from build123d import *

# Parameters (mm, degrees)
F0_W      = 31.75
F0_H      = 31.75
F1_DEPTH  = 60.33
F2_W      = 22.23
F2_H      = 22.23
F3_DEPTH  = 6.35
F4_W      = 31.75
F4_H      = 31.75
F5_DEPTH  = 112.71
F6_W      = 22.23
F6_H      = 22.23
F7_DEPTH  = 6.35
F8_W      = 31.75
F8_H      = 31.75
F8_W_2    = 22.23
F8_H_2    = 22.23
F9_DEPTH  = 112.71
F10_W     = 22.23
F10_H     = 22.23
F11_DEPTH = 6.35
F12_W     = 31.75
F12_H     = 31.75
F12_W_2   = 22.23
F12_H_2   = 22.23
F13_DEPTH = 112.71
F14_W     = 22.23
F14_H     = 22.23
F15_DEPTH = 6.35
F16_W     = 31.75
F16_H     = 31.75
F17_DEPTH = 112.71
F18_W     = 22.23
F18_H     = 22.23
F19_DEPTH = 6.35
F20_W     = 31.75
F20_H     = 31.75
F20_W_2   = 22.23
F20_H_2   = 22.23
F21_DEPTH = 112.71
F22_W     = 22.23
F22_H     = 22.23
F23_DEPTH = 6.35
F24_W     = 31.75
F24_H     = 31.75
F24_W_2   = 22.23
F24_H_2   = 22.23
F25_DEPTH = 25.4
F26_W     = 22.23
F26_H     = 22.23
F27_DEPTH = 6.35
F28_W     = 31.75
F28_H     = 31.75
F28_W_2   = 22.23
F28_H_2   = 22.23
F29_DEPTH = 31.75
F32_DEPTH = 12.7
F34_DEPTH = 12.7
F36_DEPTH = 12.7
F38_DEPTH = 12.7
F40_DEPTH = 12.7
F41_W     = 12.7
F41_H     = 12.7
F42_DEPTH = 736.6
F43_DEPTH = 6.35


with BuildPart() as f1:
    # F0 (on Top) → F1 (new body)
    with BuildSketch(Plane.XY):
        with Locations((15.875, 15.875)):
            Rectangle(F0_W, F0_H)
    extrude(amount=F1_DEPTH)

    # F2 (on face) → F3 (join)
    with BuildSketch(Plane.XY.offset(60.33)):
        with Locations((15.875, 15.875)):
            Rectangle(F2_W, F2_H)
    extrude(amount=F3_DEPTH)

    # F4 (on face) → F5 (join)
    with BuildSketch(Plane.XY.offset(66.68)):
        with Locations((15.875, 15.875)):
            Rectangle(F4_W, F4_H)
    extrude(amount=F5_DEPTH)

    # F6 (on face) → F7 (join)
    with BuildSketch(Plane.XY.offset(179.39)):
        with Locations((15.875, 15.875)):
            Rectangle(F6_W, F6_H)
    extrude(amount=F7_DEPTH)

    # F8 (on face) → F9 (join)
    with BuildSketch(Plane.XY.offset(185.74)):
        with Locations((15.875, 15.875)):
            Rectangle(F8_W, F8_H)
        with Locations((15.875, 15.875)):
            Rectangle(F8_W_2, F8_H_2, mode=Mode.SUBTRACT)
        with Locations((15.875, 15.875)):
            Rectangle(F8_W_2, F8_H_2)
    extrude(amount=F9_DEPTH)

    # F10 (on face) → F11 (join)
    with BuildSketch(Plane.XY.offset(298.45)):
        with Locations((15.875, 15.875)):
            Rectangle(F10_W, F10_H)
    extrude(amount=F11_DEPTH)

    # F12 (on face) → F13 (join)
    with BuildSketch(Plane.XY.offset(304.8)):
        with Locations((15.875, 15.875)):
            Rectangle(F12_W, F12_H)
        with Locations((15.875, 15.875)):
            Rectangle(F12_W_2, F12_H_2, mode=Mode.SUBTRACT)
        with Locations((15.875, 15.875)):
            Rectangle(F12_W_2, F12_H_2)
    extrude(amount=F13_DEPTH)

    # F14 (on face) → F15 (join)
    with BuildSketch(Plane.XY.offset(417.51)):
        with Locations((15.875, 15.875)):
            Rectangle(F14_W, F14_H)
    extrude(amount=F15_DEPTH)

    # F16 (on face) → F17 (join)
    with BuildSketch(Plane.XY.offset(423.86)):
        with Locations((15.875, 15.875)):
            Rectangle(F16_W, F16_H)
    extrude(amount=F17_DEPTH)

    # F18 (on face) → F19 (join)
    with BuildSketch(Plane.XY.offset(536.57)):
        with Locations((15.875, 15.875)):
            Rectangle(F18_W, F18_H)
    extrude(amount=F19_DEPTH)

    # F20 (on face) → F21 (join)
    with BuildSketch(Plane.XY.offset(542.92)):
        with Locations((15.875, 15.875)):
            Rectangle(F20_W, F20_H)
        with Locations((15.875, 15.875)):
            Rectangle(F20_W_2, F20_H_2, mode=Mode.SUBTRACT)
        with Locations((15.875, 15.875)):
            Rectangle(F20_W_2, F20_H_2)
    extrude(amount=F21_DEPTH)

    # F22 (on face) → F23 (join)
    with BuildSketch(Plane.XY.offset(655.63)):
        with Locations((15.875, 15.875)):
            Rectangle(F22_W, F22_H)
    extrude(amount=F23_DEPTH)

    # F24 (on face) → F25 (join)
    with BuildSketch(Plane.XY.offset(661.98)):
        with Locations((15.875, 15.875)):
            Rectangle(F24_W, F24_H)
        with Locations((15.875, 15.875)):
            Rectangle(F24_W_2, F24_H_2, mode=Mode.SUBTRACT)
        with Locations((15.875, 15.875)):
            Rectangle(F24_W_2, F24_H_2)
    extrude(amount=F25_DEPTH)

    # F26 (on face) → F27 (join)
    with BuildSketch(Plane.XY.offset(687.38)):
        with Locations((15.875, 15.875)):
            Rectangle(F26_W, F26_H)
    extrude(amount=F27_DEPTH)

    # F28 (on face) → F29 (join)
    with BuildSketch(Plane.XY.offset(693.73)):
        with Locations((15.875, 15.875)):
            Rectangle(F28_W, F28_H)
        with Locations((15.875, 15.875)):
            Rectangle(F28_W_2, F28_H_2, mode=Mode.SUBTRACT)
        with Locations((15.875, 15.875)):
            Rectangle(F28_W_2, F28_H_2)
    extrude(amount=F29_DEPTH)

    # F31 (on face) → F32 (cut)
    with BuildSketch(Plane.XZ):
        with BuildLine():
            Line((15.875, 123.035), (20.64, 123.035))
            ThreePointArc((20.64, 123.035), (12.5056361876, 126.4043638124), (15.875, 118.27))
            Line((15.875, 118.27), (15.875, 123.035))
        make_face()
        with BuildLine():
            ThreePointArc((15.875, 118.27), (19.2443638124, 119.6656361876), (20.64, 123.035))
            Line((20.64, 123.035), (15.875, 123.035))
            Line((15.875, 123.035), (15.875, 118.27))
        make_face()
    extrude(amount=-F32_DEPTH, mode=Mode.SUBTRACT)

    # F33 (on face) → F34 (cut)
    with BuildSketch(Plane.YZ.offset(31.75)):
        with BuildLine():
            Line((15.875, 242.095), (20.64, 242.095))
            ThreePointArc((20.64, 242.095), (12.5056361876, 245.4643638124), (15.875, 237.33))
            Line((15.875, 237.33), (15.875, 242.095))
        make_face()
        with BuildLine():
            ThreePointArc((15.875, 237.33), (19.2443638124, 238.7256361876), (20.64, 242.095))
            Line((20.64, 242.095), (15.875, 242.095))
            Line((15.875, 242.095), (15.875, 237.33))
        make_face()
    extrude(amount=-F34_DEPTH, mode=Mode.SUBTRACT)

    # F35 (on face) → F36 (cut)
    with BuildSketch(Plane.XZ):
        with BuildLine():
            Line((15.875, 361.155), (20.64, 361.155))
            ThreePointArc((20.64, 361.155), (12.5056361876, 364.5243638124), (15.875, 356.39))
            Line((15.875, 356.39), (15.875, 361.155))
        make_face()
        with BuildLine():
            ThreePointArc((15.875, 356.39), (19.2443638124, 357.7856361876), (20.64, 361.155))
            Line((20.64, 361.155), (15.875, 361.155))
            Line((15.875, 361.155), (15.875, 356.39))
        make_face()
    extrude(amount=-F36_DEPTH, mode=Mode.SUBTRACT)

    # F37 (on face) → F38 (cut)
    with BuildSketch(Plane.YZ.offset(31.75)):
        with BuildLine():
            Line((15.875, 480.215), (20.64, 480.215))
            ThreePointArc((20.64, 480.215), (12.5056361876, 483.5843638124), (15.875, 475.45))
            Line((15.875, 475.45), (15.875, 480.215))
        make_face()
        with BuildLine():
            ThreePointArc((15.875, 475.45), (19.2443638124, 476.8456361876), (20.64, 480.215))
            Line((20.64, 480.215), (15.875, 480.215))
            Line((15.875, 480.215), (15.875, 475.45))
        make_face()
    extrude(amount=-F38_DEPTH, mode=Mode.SUBTRACT)

    # F39 (on face) → F40 (cut)
    with BuildSketch(Plane.XZ):
        with BuildLine():
            Line((15.875, 599.275), (20.64, 599.275))
            ThreePointArc((20.64, 599.275), (12.5056361876, 602.6443638124), (15.875, 594.51))
            Line((15.875, 594.51), (15.875, 599.275))
        make_face()
        with BuildLine():
            ThreePointArc((15.875, 594.51), (19.2443638124, 595.9056361876), (20.64, 599.275))
            Line((20.64, 599.275), (15.875, 599.275))
            Line((15.875, 599.275), (15.875, 594.51))
        make_face()
    extrude(amount=-F40_DEPTH, mode=Mode.SUBTRACT)

    # F41 (on face) → F42 (cut)
    with BuildSketch(Plane.XY.offset(725.48)):
        with Locations((15.87, 15.87)):
            Rectangle(F41_W, F41_H)
    extrude(amount=-F42_DEPTH, mode=Mode.SUBTRACT)

    # F30 (on face) → F43 (cut)
    with BuildSketch(Plane(origin=(0, 0, 0), x_dir=(1, 0, 0), z_dir=(0, 0, -1))):
        with BuildLine():
            ThreePointArc((6.35, -15.875), (9.1398079092, -22.6101920908), (15.875, -25.4))
            Line((15.875, -25.4), (15.875, -15.875))
            Line((15.875, -15.875), (6.35, -15.875))
        make_face()
        with BuildLine():
            Line((15.875, -15.875), (15.875, -25.4))
            ThreePointArc((15.875, -25.4), (22.6101920908, -22.6101920908), (25.4, -15.875))
            ThreePointArc((25.4, -15.875), (15.875, -6.35), (6.35, -15.875))
            Line((6.35, -15.875), (15.875, -15.875))
        make_face()
    extrude(amount=-F43_DEPTH, mode=Mode.SUBTRACT)


solid = f1.part
Design review of the part built by this model. Coordinates are the model's own, in mm. A direction names the side the tool comes from. Coordinates: 2 decimals unless noted, no trailing zeros. Order: outer loops, then holes, each group sorted by start corner. A loop starts at its lowest first (then second) coordinate and runs counter-clockwise, first axis right, second up. Notation, with made-up numbers: M 6.25,84 L 59.25,84 A16 ccw 59.25,109 Z; hole C 1.5,24 d11. An arc over 180 degrees is marked long. Use a Markdown table: item, result.
(1) For faces 1 (the cylindrical face through (25.32, 14.64, 3.13)), 2 (the flat face through (31.75, 16, 709)), 3 (the flat face through (16, 2, 298.45)), 4 (the flat face through (22.22, 16, 371)), 5 (the flat face through (16, 31.75, 122)), list the 3-axis set-ups (+Z, -Z, +X, -X, +Y, -Y) from which the entire face can be reached by the end or side of a thin tool; tool diameter is ignored.
Worked answers:
| item | result |
|---|---|
| face 1 | -Z |
| face 2 | +Z, -Z, +X, +Y, -Y |
| face 3 | none |
| face 4 | +Z, -Z |
| face 5 | +Z, -Z, +X, -X, +Y |
(2) Draft analysis for pull direction Y (two halves, no side actions). For faces 6 (the flat face through (0, 16, 122)), 7 (the flat face through (9.52, 16, 371)), 8 (the flat face through (16, 31.75, 709)), state which applies: released by +Y, released by -Y, zero draft, split by the parting line, or undercut.
Worked answers:
| item | result |
|---|---|
| face 6 | zero draft |
| face 7 | undercut |
| face 8 | released by +Y |
(3) Wall thickness on probe 1 along X at (y, z) = (11.5, 614); probe 2 along Z at (x, y) = (19.5, 23.5): over which ranges is each line inside the solid? List them lowest first.
Worked answers:
| item | result |
|---|---|
| probe 1 | x = 0 to 9.52, 22.22 to 31.75 |
| probe 2 | z = 6.35 to 725.48 |
(4) Add section A-A (z = 318). Give the boundary of the cut face in (x, y), then the cut area to 3 significant figures.
Worked answers:
| item | result |
|---|---|
| outline | M 0,0 L 31.75,0 L 31.75,31.75 L 0,31.75 Z; hole M 9.52,9.52 L 22.22,9.52 L 22.22,22.22 L 9.52,22.22 Z |
| area | 847 mm2 |
(5) For P1, Ø8, axis at x = 17, y = 18, coming from the +Z side; P2, Ø16, axis at x = 22, y = 16.5, coming from the +Z side; P3, Ø5, axis at x = 20, y = 14, coming from the -Z side; P4, Ø3, axis at x = 17.5, z = 301, coming from the -Y side, all flat-tipped, find the tip position at first contact; note any pin that passes through.
Worked answers:
| item | result |
|---|---|
| P1 | passes through |
| P2 | stops at z = 725.48 |
| P3 | stops at z = 6.35 |
| P4 | stops at y = 4.76 |
